```python
from build123d import *

# Parameters (mm, degrees)
SKETCH_R           = 103.248116
PAD_DEPTH          = 6
SKETCH001_R        = 6
POCKET_DEPTH       = 590.183803
POLARPATTERN_COUNT = 2


with BuildPart() as part:
    # Sketch → Pad (new body)
    with BuildSketch(Plane.XY):
        Circle(SKETCH_R)
    extrude(amount=PAD_DEPTH)

    # Sketch001 (on Face3 of Pad) → Pocket (cut, through all)
    with BuildSketch(Plane.XY.offset(6)):
        with Locations((0, 50)):
            Circle(SKETCH001_R)
    pocket = extrude(amount=-POCKET_DEPTH, mode=Mode.SUBTRACT)

    # PolarPattern: Pocket ×2 about axis
    polarpattern_axis = Axis((0, 0, 6), (0, 0, 1))
    for i in range(1, POLARPATTERN_COUNT):
        add(pocket.rotate(polarpattern_axis, i * 360 / POLARPATTERN_COUNT), mode=Mode.SUBTRACT)


solid = part.part
```
CAD build for the part. Positions are in the model's coordinates, mm. Round coordinates to 2 decimals unless told otherwise and drop trailing zeros. Write each loop counter-clockwise with the first axis right and the second up, starting at its lowest first coordinate (ties: lowest second). Pieces come first, ordered by that corner, then holes. Notation, with made-up numbers: M 40.25,-14 L 77.25,-14 A13 ccw 77.25,-2 Z; hole C -7.5,53 d9. An arc over 180 degrees is marked long. One line per question, with ' | ' between items.
1. Cut at B-B on z = 4.45. Write the cut outline in (x, y).
Working result:
outline: C 0,0 d206.5; hole C 0,-50 d12; hole C 0,50 d12
2. Cut at D-D on y = -24. Write the cut outline in (x, z).
Working result:
outline: M -100.42,0 L 100.42,0 L 100.42,6 L -100.42,6 Z
3. Probe L1, parallel to Y at x = 0, z = 1.35; L2, parallel to X at y = 55.5, z = 3.9; L3, parallel to X at y = -49.5, z = 3.7. List the from-to ranges inside material, lowest first. Write a range as from..to.
Working result:
L1: -103.25..-56, -44..44, 56..103.25 | L2: -87.06..-2.4, 2.4..87.06 | L3: -90.61..-5.98, 5.98..90.61
4. Cut at C-C on y = 50. Write the cut outline in (x, z).
Working result:
outline: M -90.33,0 L -6,0 L -6,6 L -90.33,6 Z; M 6,0 L 90.33,0 L 90.33,6 L 6,6 Z
5. Pin check, flat tips, straight feed: pin 1 Ø19 at (x, y) = (0, -50) entering from -Z; pin 2 Ø3 at (y, z) = (64.5, 3) entering from -X; pin 3 Ø2 at (y, z) = (10, 1) entering from -X. Stop position of each tip, or through.
Working result:
pin 1: z = 0 | pin 2: x = -81.8 | pin 3: x = -102.86
6. Cut at A-A on x = 0. Write the cut outline in (y, z).
Working result:
outline: M -103.25,0 L -56,0 L -56,6 L -103.25,6 Z; M -44,0 L 44,0 L 44,6 L -44,6 Z; M 56,0 L 103.25,0 L 103.25,6 L 56,6 Z
7. Mould opens along X. For faces 1 (the flat face through (-1, 1, 6)), 2 (the cylindrical face through (-81.934, -62.825, 2.958)), 3 (the cylindrical face through (1.301, -44.143, 3.042)) say: pulls with the +X half, pulls with the -X half, needs draft (parallel to the pull), parting line crosses it, or undercut.
Working result:
face 1: needs draft | face 2: parting line crosses it | face 3: undercut
